from build123d import *

# Parameters (mm, degrees)
F1_DEPTH = 15
F2_DEPTH = 7.5


with BuildPart() as f1:
    # F0 (on Front) → F1 (new body, symmetric)
    with BuildSketch(Plane.XZ):
        Polygon((0, 30), (0, 0), (40, 0), (40, 15), (30, 18.75), (10, 18.75), (10, 26.25), align=None)
        Polygon((30, 18.75), (10, 26.25), (10, 18.75), align=None)
    extrude(amount=F1_DEPTH, both=True)

    # F0 (on Front) → F2 (join, symmetric)
    with BuildSketch(Plane.XZ):
        Polygon((30, 26.25), (10, 26.25), (30, 18.75), align=None)
    extrude(amount=F2_DEPTH, both=True)


solid = f1.part
Read the model definition and answer for the solid it produces. Units are mm, in the model's axes. A direction names the side the tool comes from. Coordinates: 2 decimals unless noted, no trailing zeros. Loops run counter-clockwise (first coordinate to the right, second up) from the corner with the lowest first, then second, coordinate; pieces in that order, holes last. Notation, with made-up numbers: (86, -25.5) -> (130, -25.5) arc R16 cw to (130, -7.5) -> close; hole circle Ø1 at (2, 32.25). An arc over 180 degrees is marked (long way). Answer in a Markdown table with one row per item.
Item 1: Each of these flat-tipped pins is pushed along its axis until it touches: P1, Ø1.5, axis at x = 8.5, y = -7.5, coming from the +Z side; P2, Ø2, axis at x = 8, y = -1, coming from the +Z side (3 decimals); P3, Ø16.5, axis at x = 17, y = 2, coming from the +Z side; P4, Ø12, axis at y = 6, z = 17, coming from the +X side. Where does it stop, or does it pass through?
Returned:
| item | result |
|---|---|
| P1 | stops at z = 27.09 |
| P2 | stops at z = 27.375 |
| P3 | stops at z = 26.72 |
| P4 | stops at x = 40 |
Item 2: Straight lines are drawn through the part: line 1 along X through (y, z) = (5.25, 24.5); line 2 along Z through (x, y) = (11, -3); line 3 along Y through (x, z) = (22, 23.25). For each, find the intervals that lie inside material, in ascending order. Write a range as [from, to].
Returned:
| item | result |
|---|---|
| line 1 | x = [0, 30] |
| line 2 | z = [0, 26.25] |
| line 3 | y = [-7.5, 7.5] |
Item 3: A cutting plane is placed at B-B on x = 16. Determine the outline of the cut face in (y, z).
Returned:
| item | result |
|---|---|
| outline | (-15, 0) -> (15, 0) -> (15, 24) -> (7.5, 24) -> (7.5, 26.25) -> (-7.5, 26.25) -> (-7.5, 24) -> (-15, 24) -> close |
Item 4: A cutting plane is placed at C-C on y = -0.5. Determine the outline of the cut face in (x, z).
Returned:
| item | result |
|---|---|
| outline | (0, 0) -> (40, 0) -> (40, 15) -> (30, 18.75) -> (30, 26.25) -> (10, 26.25) -> (0, 30) -> close |
Item 5: A cutting plane is placed at A-A on z = 20.25. Determine the outline of the cut face in (x, y).
Returned:
| item | result |
|---|---|
| outline | (0, -15) -> (26, -15) -> (26, -7.5) -> (30, -7.5) -> (30, 7.5) -> (26, 7.5) -> (26, 15) -> (0, 15) -> close |
Item 6: A cutting plane is placed at D-D on z = 15.75. Determine the outline of the cut face in (x, y), plus the area to 3 significant figures.
Returned:
| item | result |
|---|---|
| outline | (0, -15) -> (38, -15) -> (38, 15) -> (0, 15) -> close |
| area | 1,140 mm^2 |
Item 7: For faces 1 (the flat face through (24, 7.5, 24)), 2 (the flat face through (20, 0, 26.25)), 3 (the flat face through (0, 0, 15)), 4 (the flat face through (20, -15, 12)), 5 (the flat face through (24, -7.5, 24)), determine the directions among +Z, -Z, +X, -X, +Y, -Y from which every point of the face is accessible in a straight line to the end or side of a thin tool.
Returned:
| item | result |
|---|---|
| face 1 | +Z, +X, +Y |
| face 2 | +Z, +X, +Y, -Y |
| face 3 | +Z, -Z, -X, +Y, -Y |
| face 4 | +Z, -Z, +X, -X, -Y |
| face 5 | +Z, +X, -Y |
